Geometry check sheet. Reference: the model listing, model coordinates, mm. Face numbers are marked on the shaded views. A direction names the side the tool comes from. Give positions to 0.01 mm unless a question says otherwise; leave off trailing zeros. Loops run counter-clockwise (first coordinate to the right, second up) from the corner with the lowest first, then second, coordinate; pieces in that order, holes last. Notation, with made-up numbers: (30.5, 85.5) -> (36.5, 85.5) arc R25 cw to (36.5, 97.5) -> close; hole circle Ø10 at (2.5, -32.5). An arc over 180 degrees is marked (long way). One line per question, with ' | ' between items.
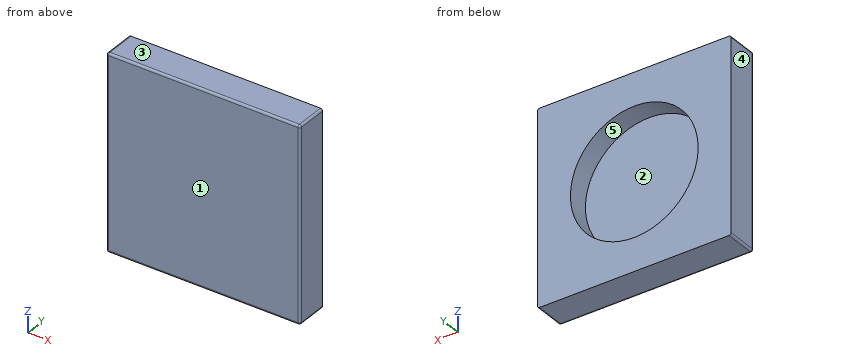
from build123d import *

# Parameters (mm, degrees)
SKETCH1_W           = 45.5
SKETCH1_H           = 45.5
BOSS_EXTRUDE1_DEPTH = 7.5
FILLET1_R           = 0.5
SKETCH2_R           = 15
CUT_EXTRUDE1_DEPTH  = 5


with BuildPart() as part:
    # Sketch1 → Boss-Extrude1 (new body)
    with BuildSketch(Plane(origin=(0, 0, 0), x_dir=(1, 0, 0), z_dir=(0, 1, 0))):
        Rectangle(SKETCH1_W, SKETCH1_H)
    extrude(amount=BOSS_EXTRUDE1_DEPTH)

    # Fillet1
    fillet1_edges = [part.edges().sort_by_distance(p)[0] for p in [
        (0, 0, 22.75),
        (-22.75, 0, 0),
        (0, 0, -22.75),
        (22.75, 0, 0),
        (22.75, 3.75, 22.75),
        (-22.75, 3.75, 22.75),
        (-22.75, 3.75, -22.75),
        (22.75, 3.75, -22.75),
    ]]
    fillet(fillet1_edges, radius=FILLET1_R)

    # Sketch2 → Cut-Extrude1 (cut)
    with BuildSketch(Plane(origin=(0, 7.5, 0), x_dir=(1, 0, 0), z_dir=(0, 1, 0))):
        Circle(SKETCH2_R)
    extrude(amount=-CUT_EXTRUDE1_DEPTH, mode=Mode.SUBTRACT)


solid = part.part
Item 1: Sectioned sample at C-C (z = 0). Record the cut outline in (x, y).
Result:
outline: (-22.75, 0.5) arc R0.5 ccw to (-22.25, 0) -> (22.25, 0) arc R0.5 ccw to (22.75, 0.5) -> (22.75, 7.5) -> (15, 7.5) -> (15, 2.5) -> (-15, 2.5) -> (-15, 7.5) -> (-22.75, 7.5) -> close
Item 2: Set-up check for the marked faces 4 and 5: record each of +Z, -Z, +X, -X, +Y, -Y from which the full face is reachable in a straight line by a thin tool's end or side.
Result:
face 4: +Z, -Z, -X, +Y, -Y | face 5: +Y
Item 3: Sectioned sample at A-A (y = 5.75). Record the cut outline in (x, z).
Result:
outline: (-22.75, -22.25) arc R0.5 ccw to (-22.25, -22.75) -> (22.25, -22.75) arc R0.5 ccw to (22.75, -22.25) -> (22.75, 22.25) arc R0.5 ccw to (22.25, 22.75) -> (-22.25, 22.75) arc R0.5 ccw to (-22.75, 22.25) -> close; hole circle Ø30 at (0, 0)
Item 4: Scan lines: probe 1 along Z at (x, y) = (0, 6.2); probe 2 along X at (y, z) = (5, 6.5). Record each from-to range of solid material in increasing order.
Result:
probe 1: -22.75 to -15, 15 to 22.75 | probe 2: -22.75 to -13.52, 13.52 to 22.75
Item 5: Release check for a two-part mould opening along Z. For the marked faces 1, 2 and 3 record: pulls with the +Z half, pulls with the -Z half, needs draft (parallel to the pull), parting line crosses it, or undercut.
Result:
face 1: needs draft | face 2: undercut | face 3: pulls with the +Z half
Item 6: Depth check by flat-ended pin: pin 1 Ø5 at (x, z) = (-5, 6) entering from +Y. Enter the tip coordinate at first touch or a pass-through.
Result:
pin 1: y = 2.5
Item 7: Sectioned sample at B-B (x = 0). Record the cut outline in (y, z).
Result:
outline: (0, -22.25) arc R0.5 ccw to (0.5, -22.75) -> (7.5, -22.75) -> (7.5, -15) -> (2.5, -15) -> (2.5, 15) -> (7.5, 15) -> (7.5, 22.75) -> (0.5, 22.75) arc R0.5 ccw to (0, 22.25) -> close
